The listing builds one solid part. Answer for the finished solid, in the listing's coordinates (mm). Face numbers are marked on the shaded views. Give positions to 0.01 mm unless a question says otherwise; leave off trailing zeros. Write each loop counter-clockwise with the first axis right and the second up, starting at its lowest first coordinate (ties: lowest second). Pieces come first, ordered by that corner, then holes. Notation, with made-up numbers: (49, 64) -> (97, 64) arc R20 ccw to (97, 83) -> close; hole circle Ø9 at (51, 77.5). An arc over 180 degrees is marked (long way). Put each result on its own line as item: value. Start each with the question number.
1) A cutting plane is placed at A-A (x = 54.7). Write down the section's boundary in (y, z).
2) For a pull along Y with two mould halves and no side action, classify the marked faces 1, 2, 3 and 4 as released by +Y, released by -Y, zero draft, split by the parting line, or undercut.
3) A cutting plane is placed at C-C (y = -1.5). Write down the section's boundary in (x, z), then the cut area to 3 significant figures.
4) Find the intervals of material crossed by line 1 along X through (y, z) = (6.75, -16.75); line 2 along Z through (x, y) = (60.75, -1); line 3 along Z through (x, y) = (57, 1.5), in increasing order. Write a range as from..to.
5) A cutting plane is placed at D-D (x = 58.5). Write down the section's boundary in (y, z), then the cut area to 3 significant figures.
6) A cutting plane is placed at B-B (z = -10.5). Write down the section's boundary in (x, y).
7) Flat-ended cylindrical pins translate along their axes: pin 1 Ø1 at (x, z) = (59, -14.5) entering from -Y; pin 2 Ø5 at (x, y) = (51, 3.5) entering from -Z; pin 3 Ø5 at (x, y) = (53.5, 8.5) entering from -Z. Find the tip coordinate at first contact, or state that the pin passes through.
from build123d import *

# Parameters (mm, degrees)
SKETCH016_R               = 1
PAD014_DEPTH              = 11.5
FUSION006_PLACEMENT_ANGLE = 90


with BuildPart() as sphere:
    # Sphere → Sphere (revolve)
    with BuildSketch(Plane(origin=(56.3, 0, -9), x_dir=(1, 0, 0), z_dir=(0, -1, 0))):
        with BuildLine():
            ThreePointArc((0, -6), (6, 0), (0, 6))
            Line((0, 6), (0, -6))
        make_face()
    revolve(axis=Axis((56.3, 0, -9), (0, 0, 1)))


with BuildPart() as casterwheel:
    # Sketch016 → Pad014 (new body)
    with BuildSketch(Plane.XY):
        with BuildLine():
            ThreePointArc((48.919965, -3), (56.336164, -8), (63.752362, -3))
            Line((63.752362, -3), (64.340191, -3))
            ThreePointArc((64.340191, -3), (67.34019, 0.002014), (64.336164, 2.999997))
            Line((63.752363, 2.999997), (64.336164, 2.999997))
            ThreePointArc((63.752363, 2.999997), (56.336165, 8), (48.919965, 3))
            Line((48.336164, 3), (48.919965, 3))
            ThreePointArc((48.336164, 3), (45.336163, 0), (48.336163, -3))
            Line((48.336163, -3), (48.919965, -3))
        make_face()
        with Locations((48.836164, 0)):
            Circle(SKETCH016_R, mode=Mode.SUBTRACT)
        with Locations((63.836164, 0)):
            Circle(SKETCH016_R, mode=Mode.SUBTRACT)
    extrude(amount=-PAD014_DEPTH)

    # Fusion006: union Sphere
    add(sphere.part)


with BuildPart() as casterwheel_1:
    # Fusion006 placement: moved
    add(casterwheel.part.moved(Location((54.7, -56.5, -8))).rotate(Axis((54.7, -56.5, -8), (0, 0, 1)), FUSION006_PLACEMENT_ANGLE))


solid = casterwheel_1.part
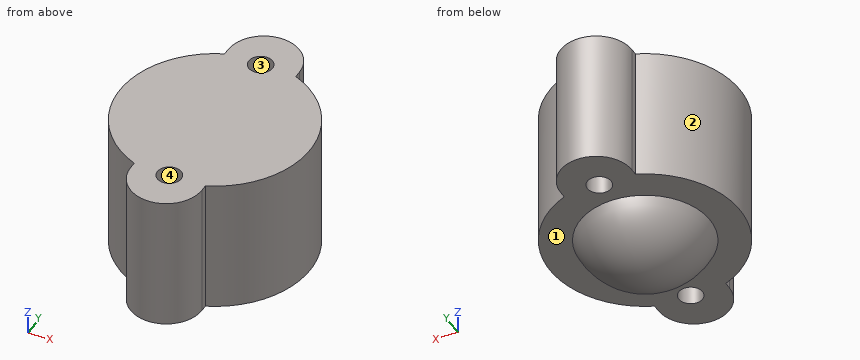
Reply:
1. outline: (-11.16, -19.5) -> (-8.66, -19.5) -> (-8.66, -8) -> (-11.16, -8) -> close; (-6.66, -19.5) -> (-5.65, -19.5) arc R6 ccw to (5.25, -19.5) -> (6.34, -19.5) -> (6.34, -8) -> (-6.66, -8) -> close; (8.34, -19.5) -> (10.84, -19.5) -> (10.84, -8) -> (8.34, -8) -> close
2. face 1: zero draft
2. face 2: split by the parting line
2. face 3: undercut
2. face 4: undercut
3. outline: (46.81, -19.5) -> (49.4, -19.5) arc R5.86 ccw to (60, -19.5) -> (62.59, -19.5) -> (62.59, -8) -> (46.81, -8) -> close
3. area: 207 mm2
4. line 1: x = 50.68..53.89, 55.51..58.72
4. line 2: z = -19.5..-8
4. line 3: z = -22.27..-8
5. outline: (-7.2, -19.5) -> (-4.11, -19.5) arc R4.64 ccw to (3.71, -19.5) -> (6.88, -19.5) -> (6.88, -8) -> (-7.2, -8) -> close
5. area: 174 mm2
6. outline: (51.7, -8.16) arc R3 ccw to (57.7, -8.16) -> (57.7, -7.58) arc R8 ccw to (57.7, 7.25) -> (57.7, 7.84) arc R3 ccw to (51.7, 7.84) -> (51.7, 7.25) arc R8 ccw to (51.7, -7.58) -> close; hole circle Ø2 at (54.7, -7.66); hole circle Ø2 at (54.7, 7.34)
7. pin 1: stops at y = -7.2
7. pin 2: stops at z = -22.34
7. pin 3: stops at z = -19.5
